Part model, mm, in its own coordinate system. A direction names the side the tool comes from. Round coordinates to 2 decimals unless told otherwise and drop trailing zeros. Loops run counter-clockwise (first coordinate to the right, second up) from the corner with the lowest first, then second, coordinate; pieces in that order, holes last. Notation, with made-up numbers: M -10,52 L 31,52 A28 ccw 31,73 Z; hole C 43,66 d10. An arc over 180 degrees is marked long. Put each result on its own line as item: value. Start each with the question number.
1) Slice it at D-D on z = 22. Give the cut face in (x, y), then the cut area to 3 significant figures.
2) Probe line 1 along X through (y, z) = (5.5, 0); line 2 along X through (y, z) = (9.85, 0); line 3 along Z through (x, y) = (19.5, 6.5). List the from-to ranges inside material, lowest first.
3) Which spindle directions (+Z, -Z, +X, -X, +Y, -Y) get a long thin tool onto all of the face, cutting with end or side? Do faces 4 (the cylindrical face through (-6.31, 10.57, -20.03)), 5 (the cylindrical face through (15.88, 4.04, 17.32)), 6 (the flat face through (-22, 9, 13)). Say none if no direction does.
4) Pull direction Z, two halves, no side cores. Call faces 1 (the cylindrical face through (28.75, 6.41, 6.38)), 2 (the cylindrical face through (0.106, 10.774, -27.623)), 3 (the flat face through (13, 13, -17)): +Z half, -Z half, draft (parallel to the pull), parting line (faces both ways), or undercut.
5) Slice it at A-A on z = -6. Give the cut face in (x, y).
6) Slice it at C-C on y = 3.5. Give the cut face in (x, z).
7) Slice it at B-B on x = -10. Give the cut face in (y, z).
8) Drop flat-ended pins along their axis: pin 1 Ø2.5 at (x, z) = (0.5, -26.5) entering from +Y; pin 2 Ø1 at (x, y) = (22.5, 6.5) entering from -Z; pin 3 Ø5 at (y, z) = (2, -13) entering from -X. Give the stop position or say it passes through.
```python
from build123d import *

# Parameters (mm, degrees)
SKETCH1_R           = 29.45
SKETCH1_R_2         = 21
BOSS_EXTRUDE1_DEPTH = 13
SKETCH2_R           = 2.4
CUT_EXTRUDE1_DEPTH  = 4
CHAMFER1_SIZE       = 0.5
SKETCH4_R           = 23.5
CUT_EXTRUDE2_DEPTH  = 8.2


with BuildPart() as part:
    # Sketch1 → Boss-Extrude1 (new body)
    with BuildSketch(Plane(origin=(0, 0, 0), x_dir=(1, 0, 0), z_dir=(0, 1, 0))):
        with Locations(Location((0, 0, 0), (0, 0, 90))):
            Circle(SKETCH1_R)
        with Locations(Location((0, 0, 0), (0, 0, 90))):
            Circle(SKETCH1_R_2, mode=Mode.SUBTRACT)
    extrude(amount=BOSS_EXTRUDE1_DEPTH)

    # Sketch2 → Cut-Extrude1 (cut)
    with BuildSketch(Plane(origin=(0, 13, 0), x_dir=(1, 0, 0), z_dir=(0, 1, 0))):
        with Locations(Location((0, 25.225, 0), (0, 0, 270))):
            Circle(SKETCH2_R)
        with Locations(Location((21.84549081, -12.6125, 0), (0, 0, 270))):
            Circle(SKETCH2_R)
        with Locations(Location((-21.84549081, -12.6125, 0), (0, 0, 270))):
            Circle(SKETCH2_R)
    extrude(amount=-CUT_EXTRUDE1_DEPTH, mode=Mode.SUBTRACT)

    # Chamfer1
    chamfer1_edges = [part.edges().sort_by_distance(p)[0] for p in [
        (0, 13, -27.625),
        (21.84549081, 13, 10.2125),
        (-21.84549081, 13, 10.2125),
    ]]
    chamfer(chamfer1_edges, length=CHAMFER1_SIZE)

    # Sketch4 → Cut-Extrude2 (cut)
    with BuildSketch(Plane.XZ):
        with Locations(Location((0, 0, 0), (0, 0, 270))):
            Circle(SKETCH4_R)
    extrude(amount=-CUT_EXTRUDE2_DEPTH, mode=Mode.SUBTRACT)


solid = part.part
```
Recorded:
1. outline: M -19.58,0 L -8.26,0 L -8.26,8.2 L 8.26,8.2 L 8.26,0 L 19.58,0 L 19.58,13 L -19.58,13 Z
1. area: 374 mm2
2. line 1: x = -29.45 to -23.5, 23.5 to 29.45
2. line 2: x = -29.45 to -21, 21 to 29.45
2. line 3: z = -22.07 to -13.11, 13.11 to 22.07
3. face 4: +Y, -Y
3. face 5: -Y
3. face 6: +Y
4. face 1: parting line
4. face 2: undercut
4. face 3: draft
5. outline: M -28.83,0 L -22.72,0 L -22.72,8.2 L -20.12,8.2 L -20.12,13 L -28.83,13 Z; M 20.12,8.2 L 22.72,8.2 L 22.72,0 L 28.83,0 L 28.83,13 L 20.12,13 Z
6. outline: C 0,0 d58.9; hole C 0,0 d47
7. outline: M 0,-27.7 L 13,-27.7 L 13,-18.47 L 8.2,-18.47 L 8.2,-21.27 L 0,-21.27 Z; M 0,21.27 L 8.2,21.27 L 8.2,18.47 L 13,18.47 L 13,27.7 L 0,27.7 Z
8. pin 1: stops at y = 12.72
8. pin 2: stops at z = -19.58
8. pin 3: stops at x = -27.51
